Build history of the part. All positions in model axes, mm. A direction names the side the tool comes from. Round coordinates to 2 decimals unless told otherwise and drop trailing zeros. Loops run counter-clockwise (first coordinate to the right, second up) from the corner with the lowest first, then second, coordinate; pieces in that order, holes last. Notation, with made-up numbers: (42.25, 6) - (92.25, 6) arc R14 cw to (92.25, 20) - close; hole circle Ø9 at (-10.5, 21.5). An arc over 180 degrees is marked (long way). Use a Markdown table: item, result.
from build123d import *

# Parameters (mm, degrees)
SKETCH1_W           = 62
SKETCH1_H           = 33
BOSS_EXTRUDE1_DEPTH = 20
SHELL1_T            = -2
SKETCH2_W           = 4
SKETCH2_H           = 5
BOSS_EXTRUDE2_DEPTH = 123
SKETCH3_W           = 5
SKETCH3_H           = 5
BOSS_EXTRUDE3_DEPTH = 53
SKETCH4_W           = 5
SKETCH4_H           = 4.999777887
BOSS_EXTRUDE4_DEPTH = 53
SKETCH5_R           = 1.5
CUT_EXTRUDE1_DEPTH  = 53
SKETCH6_R           = 1.1
CUT_EXTRUDE2_DEPTH  = 10


with BuildPart() as part:
    # Sketch1 → Boss-Extrude1 (new body)
    with BuildSketch(Plane.XY):
        Rectangle(SKETCH1_W, SKETCH1_H)
    extrude(amount=BOSS_EXTRUDE1_DEPTH)

    # Shell1
    shell1_openings = [part.faces().sort_by_distance(p)[0] for p in [
        (0, 0, 20),
    ]]
    offset(amount=SHELL1_T, openings=shell1_openings, kind=Kind.INTERSECTION)

    # Sketch2 → Boss-Extrude2 (add)
    with BuildSketch(Plane(origin=(0, 16.5, 0), x_dir=(1, 0, 0), z_dir=(0, 1, 0))):
        with Locations((-28, -4.324522586)):
            Rectangle(SKETCH2_W, SKETCH2_H)
        with Locations((28, -4.324522586)):
            Rectangle(SKETCH2_W, SKETCH2_H)
    extrude(amount=BOSS_EXTRUDE2_DEPTH)

    # Sketch3 → Boss-Extrude3 (add)
    with BuildSketch(Plane(origin=(-26, 0, 0), x_dir=(0, 0, -1), z_dir=(1, 0, 0))):
        with Locations((-4.324522586, 66.417337004)):
            Rectangle(SKETCH3_W, SKETCH3_H)
    extrude(amount=BOSS_EXTRUDE3_DEPTH)

    # Sketch4 → Boss-Extrude4 (add)
    with BuildSketch(Plane(origin=(-26, 0, 0), x_dir=(0, 0, -1), z_dir=(1, 0, 0))):
        with Locations((-4.324522586, 137.000111057)):
            Rectangle(SKETCH4_W, SKETCH4_H)
    extrude(amount=BOSS_EXTRUDE4_DEPTH)

    # Sketch5 → Cut-Extrude1 (cut)
    with BuildSketch(Plane.XY.offset(6.824522586)):
        with Locations((-27.588179803, 137.122373113)):
            Circle(SKETCH5_R)
        with Locations((27.802254523, 137.122373113)):
            Circle(SKETCH5_R)
    extrude(amount=-CUT_EXTRUDE1_DEPTH, mode=Mode.SUBTRACT)

    # Sketch6 → Cut-Extrude2 (cut)
    with BuildSketch(Plane(origin=(0, 0, 0), x_dir=(-1, 0, 0), z_dir=(0, 0, -1))):
        with Locations((-18.21842794, 9.95930811)):
            Circle(SKETCH6_R)
        with Locations((-18.21842794, -10.04069189)):
            Circle(SKETCH6_R)
        with Locations((16.78157206, -10.04069189)):
            Circle(SKETCH6_R)
        with Locations((16.78157206, 9.95930811)):
            Circle(SKETCH6_R)
    extrude(amount=-CUT_EXTRUDE2_DEPTH, mode=Mode.SUBTRACT)


solid = part.part
Q1. Pull direction Y, two halves, no side cores. Call faces 1 (the face through (-29, 0, 11)), 2 (the face through (0, -16.5, 10)), 3 (the face through (0, 63.917, 4)), 4 (the face through (-2, -15, 20)): pulls with the +Y half, pulls with the -Y half, needs draft (parallel to the pull), parting line crosses it, or undercut.
Results found:
| item | result |
|---|---|
| face 1 | undercut |
| face 2 | pulls with the -Y half |
| face 3 | undercut |
| face 4 | needs draft |
Q2. Probe line 1 (Y direction, x = -17.5, z = 3.5); line 2 (Y direction, x = -11.5, z = 12.5); line 3 (X direction, y = 69, z = 4.25). List the from-to ranges inside material, lowest first.
Results found:
| item | result |
|---|---|
| line 1 | y = -16.5 to -14.5, 14.5 to 16.5, 63.92 to 68.92, 134.5 to 139.5 |
| line 2 | y = -16.5 to -14.5, 14.5 to 16.5 |
| line 3 | x = -30 to -26, 26 to 30 |
Q3. Cut at A-A, the plane x = 9. List the corners of the cut face in (y, z).
Results found:
| item | result |
|---|---|
| outline | (-16.5, 0) - (16.5, 0) - (16.5, 20) - (14.5, 20) - (14.5, 2) - (-14.5, 2) - (-14.5, 20) - (-16.5, 20) - close; (63.92, 1.82) - (68.92, 1.82) - (68.92, 6.82) - (63.92, 6.82) - close; (134.5, 1.82) - (139.5, 1.82) - (139.5, 6.82) - (134.5, 6.82) - close |
Q4. Cut at D-D, the plane z = 5. List the corners of the cut face in (x, y).
Results found:
| item | result |
|---|---|
| outline | (-31, -16.5) - (31, -16.5) - (31, 16.5) - (30, 16.5) - (30, 139.5) - (-30, 139.5) - (-30, 16.5) - (-31, 16.5) - close; hole circle Ø3 at (-27.59, 137.12); hole (-29, -14.5) - (29, -14.5) - (29, 14.5) - (-29, 14.5) - close; hole (-26, 16.5) - (26, 16.5) - (26, 63.92) - (-26, 63.92) - close; hole (-26, 68.92) - (26, 68.92) - (26, 134.5) - (-26, 134.5) - close; hole circle Ø3 at (27.8, 137.12) |
Q5. Which spindle directions (+Z, -Z, +X, -X, +Y, -Y) get a long thin tool onto all of the face, cutting with end or side? Do faces 5 (the face through (-30, 77, 4)), 6 (the face through (29, 0, 11)), 7 (the face through (26, 40, 4)). Say none if no direction does.
Results found:
| item | result |
|---|---|
| face 5 | +Z, -Z, -X, +Y |
| face 6 | +Z |
| face 7 | +Z, -Z |
Q6. Cut at B-B, the plane y = 80. List the corners of the cut face in (x, z), plus the area to 3 significant figures.
Results found:
| item | result |
|---|---|
| outline | (-30, 1.82) - (-26, 1.82) - (-26, 6.82) - (-30, 6.82) - close; (26, 1.82) - (30, 1.82) - (30, 6.82) - (26, 6.82) - close |
| area | 40.0 mm2 |
Q7. Cut at C-C, the plane z = 13.5. List the corners of the cut face in (x, y).
Results found:
| item | result |
|---|---|
| outline | (-31, -16.5) - (31, -16.5) - (31, 16.5) - (-31, 16.5) - close; hole (-29, -14.5) - (29, -14.5) - (29, 14.5) - (-29, 14.5) - close |
Q8. Drop flat-ended pins along their axis: pin 1 (5.5 mm diameter, centred on y = 106, z = 4, fed in from -X); pin 2 (18 mm diameter, centred on x = -10, y = 68, fed in from -Z); pin 3 (2.5 mm diameter, centred on y = 95.5, z = 5, fed in from +X). Give the stop position or say it passes through.
Results found:
| item | result |
|---|---|
| pin 1 | stops at x = -30 |
| pin 2 | stops at z = 1.82 |
| pin 3 | stops at x = 30 |
